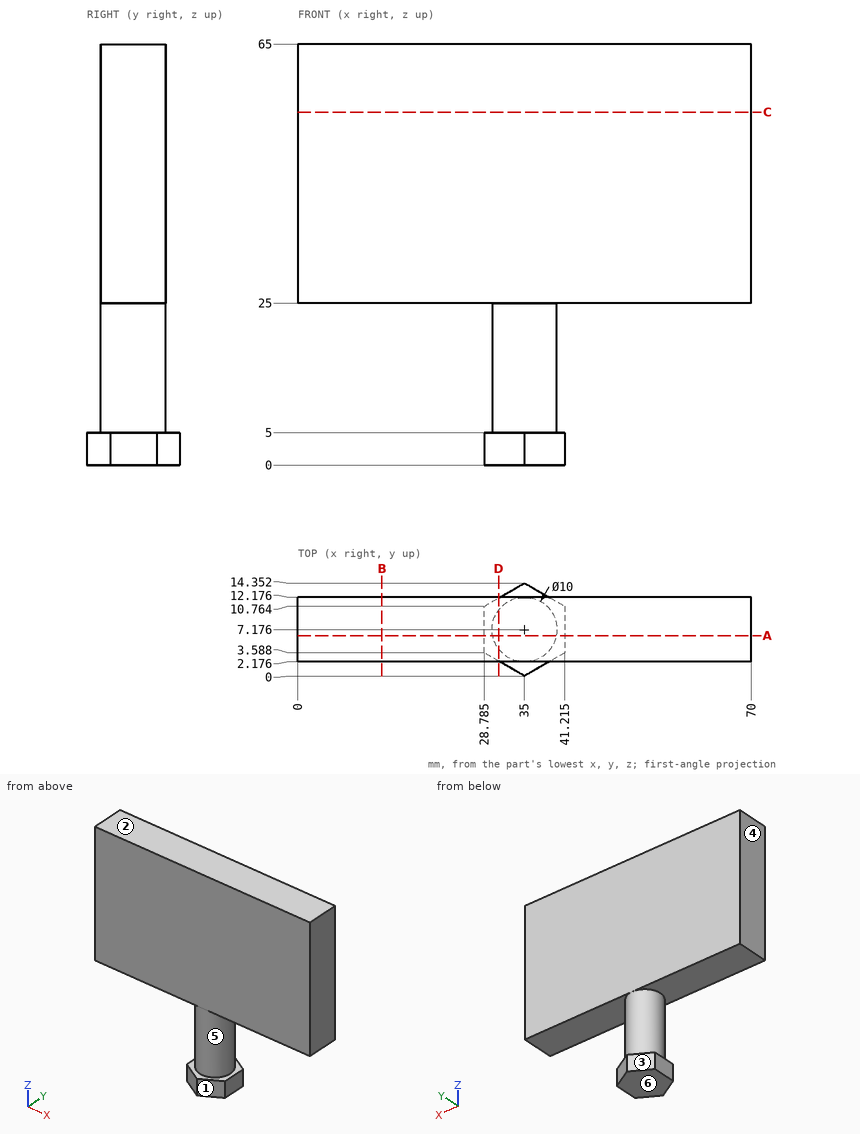
Answer from the drawing. Dimensions are ordinates in mm from the lowest x, y and z of the part. A direction names the side the tool comes from. Give positions to 0.01 mm unless a question says otherwise; leave off trailing zeros. Write each loop counter-clockwise with the first axis right and the second up, starting at its lowest first coordinate (ties: lowest second). Pieces come first, ordered by that corner, then holes. Notation, with made-up numbers: (74, -18) - (132, -18) arc R30 ccw to (132, 5) - close; hole circle Ø5 at (60.25, -6.75). An arc over 180 degrees is marked (long way). One line per item, written item: value. Start each with the question number.
1. Consider probe 1 along Z at (x, y) = (37, 2.5); probe 2 along Y at (x, z) = (46, 52); probe 3 along Z at (x, y) = (15, 4.75). Determine where each line is inside the solid, lowest interval first.
2. Find section B-B (x = 13). Write down the section's boundary in (y, z), then the cut area to 3 significant figures.
3. Given pin 1 (4 mm diameter, centred on y = 10.5, z = 10, fed in from -X); pin 2 (1.5 mm diameter, centred on y = 6.5, z = 2.5, fed in from -X) (1 decimal); pin 3 (1.5 mm diameter, centred on y = 6.5, z = 3.5, fed in from +X) (1 decimal); pin 4 (8 mm diameter, centred on y = 11.5, z = 49.5, fed in from -X), each flat-ended and moving along its own axis, determine where each tip first touches the part or whether it passes through.
4. Find section C-C (z = 54.5). Write down the section's boundary in (x, y).
5. For the marked faces 1, 2 and 3, determine the directions among +Z, -Z, +X, -X, +Y, -Y from which every point of the face is accessible in a straight line to the end or side of a thin tool.
6. Find section A-A (y = 6.25). Write down the section's boundary in (x, z) (1 decimal), then the cut area to 3 significant figures.
7. Find section D-D (x = 31). Write down the section's boundary in (y, z), then the cut area to 3 significant figures.
8. For a pull along Z with two mould halves and no side action, classify the marked faces 4, 5 and 6 as +Z half, -Z half, draft (parallel to the pull), parting line (faces both ways), or undercut.
Geometry results:
1. probe 1: 0 to 5, 25 to 65
1. probe 2: 2.18 to 12.18
1. probe 3: 25 to 65
2. outline: (2.18, 25) - (12.18, 25) - (12.18, 65) - (2.18, 65) - close
2. area: 400 mm2
3. pin 1: x = 30.18
3. pin 2: x = 28.8
3. pin 3: x = 41.2
3. pin 4: x = 0
4. outline: (0, 2.18) - (70, 2.18) - (70, 12.18) - (0, 12.18) - close
5. face 1: -Z, +X, -Y
5. face 2: +Z, +X, -X, +Y, -Y
5. face 3: -Z, -X, +Y
6. outline: (0, 25) - (30.1, 25) - (30.1, 5) - (28.8, 5) - (28.8, 0) - (41.2, 0) - (41.2, 5) - (39.9, 5) - (39.9, 25) - (70, 25) - (70, 65) - (0, 65) - close
6. area: 3,060 mm2
7. outline: (2.18, 25) - (4.18, 25) - (4.18, 5) - (2.31, 5) - (2.31, 0) - (12.04, 0) - (12.04, 5) - (10.18, 5) - (10.18, 25) - (12.18, 25) - (12.18, 65) - (2.18, 65) - close
7. area: 569 mm2
8. face 4: draft
8. face 5: undercut
8. face 6: -Z half
